```python
from build123d import *

# Parameters (mm, degrees)
ESQUISSE1_R        = 3.5
BOSS_EXTRU_1_DEPTH = 2
BOSS_EXTRU_2_START = 2
BOSS_EXTRU_2_DEPTH = 4
CONG_1_R           = 1


with BuildPart() as part:
    # Esquisse1 → Boss.-Extru.1 (new body)
    with BuildSketch(Plane.XY):
        with BuildLine():
            Line((8.486931566, 0), (59.535501901, 0))
            ThreePointArc((59.535501901, 0), (65.701431316, -2.44398639), (68.518594603, -8.448596789))
            Line((68.518594603, -8.448596789), (73.575299132, -90.829048435))
            ThreePointArc((73.575299132, -90.829048435), (76.596287018, -97.01955194), (83.109795045, -99.260737926))
            Line((83.109795045, -99.260737926), (85.106037868, -99.13820388))
            ThreePointArc((85.106037868, -99.13820388), (91.296541372, -96.117215994), (93.537727359, -89.603707966))
            Line((93.537727359, -89.603707966), (87.328590379, 11.551403211))
            ThreePointArc((87.328590379, 11.551403211), (84.511427092, 17.55601361), (78.345497677, 20))
            Line((78.345497677, 20), (-10.372916358, 20))
            ThreePointArc((-10.372916358, 20), (-16.547500996, 17.547862594), (-19.357434532, 11.527667678))
            Line((-19.357434532, 11.527667678), (-25.311005353, -89.842886985))
            ThreePointArc((-25.311005353, -89.842886985), (-23.052618299, -96.350450996), (-16.854154857, -99.355072837))
            Line((-16.854154857, -99.355072837), (-14.857595263, -99.472332322))
            ThreePointArc((-14.857595263, -99.472332322), (-8.350031252, -97.213945268), (-5.34540941, -91.015481826))
            Line((-5.34540941, -91.015481826), (-0.497586608, -8.472332322))
            ThreePointArc((-0.497586608, -8.472332322), (2.312346928, -2.452137406), (8.486931566, 0))
        make_face()
        with Locations((33.998753696, 10)):
            Circle(ESQUISSE1_R, mode=Mode.SUBTRACT)
    extrude(amount=BOSS_EXTRU_1_DEPTH)

    # Esquisse1<4> → Boss.-Extru.2 (add)
    with BuildSketch(Plane.XY.offset(BOSS_EXTRU_2_START)):
        with BuildLine():
            Line((8.486931566, 0), (59.535501901, 0))
            ThreePointArc((59.535501901, 0), (65.701431316, -2.44398639), (68.518594603, -8.448596789))
            Line((68.518594603, -8.448596789), (73.575299132, -90.829048435))
            ThreePointArc((73.575299132, -90.829048435), (76.596287018, -97.01955194), (83.109795045, -99.260737926))
            Line((83.109795045, -99.260737926), (85.106037868, -99.13820388))
            ThreePointArc((85.106037868, -99.13820388), (91.296541372, -96.117215994), (93.537727359, -89.603707966))
            Line((93.537727359, -89.603707966), (87.328590379, 11.551403211))
            ThreePointArc((87.328590379, 11.551403211), (84.511427092, 17.55601361), (78.345497677, 20))
            Line((78.345497677, 20), (-10.372916358, 20))
            ThreePointArc((-10.372916358, 20), (-16.547500996, 17.547862594), (-19.357434532, 11.527667678))
            Line((-19.357434532, 11.527667678), (-25.311005353, -89.842886985))
            ThreePointArc((-25.311005353, -89.842886985), (-23.052618299, -96.350450996), (-16.854154857, -99.355072837))
            Line((-16.854154857, -99.355072837), (-14.857595263, -99.472332322))
            ThreePointArc((-14.857595263, -99.472332322), (-8.350031252, -97.213945268), (-5.34540941, -91.015481826))
            Line((-5.34540941, -91.015481826), (-0.497586608, -8.472332322))
            ThreePointArc((-0.497586608, -8.472332322), (2.312346928, -2.452137406), (8.486931566, 0))
        make_face()
        with BuildLine():
            Line((-10.372916358, 18), (78.345497677, 18))
            ThreePointArc((78.345497677, 18), (83.141220555, 16.099121696), (85.332347556, 11.428869164))
            Line((85.332347556, 11.428869164), (91.541484536, -89.726242013))
            ThreePointArc((91.541484536, -89.726242013), (89.79833988, -94.792303812), (84.983503821, -97.141961057))
            Line((84.983503821, -97.141961057), (82.987260998, -97.264495104))
            ThreePointArc((82.987260998, -97.264495104), (77.921199199, -95.521350447), (75.571541954, -90.706514388))
            Line((75.571541954, -90.706514388), (70.514837426, -8.326062742))
            ThreePointArc((70.514837426, -8.326062742), (67.071637853, -0.987094477), (59.535501901, 2))
            Line((59.535501901, 2), (8.486931566, 2))
            ThreePointArc((8.486931566, 2), (0.940217009, -0.997056829), (-2.494146203, -8.355072837))
            Line((-2.494146203, -8.355072837), (-7.341969005, -90.898222342))
            ThreePointArc((-7.341969005, -90.898222342), (-9.678897103, -95.719249463), (-14.740335779, -97.475772727))
            Line((-14.740335779, -97.475772727), (-16.736895373, -97.358513243))
            ThreePointArc((-16.736895373, -97.358513243), (-21.557922495, -95.021585145), (-23.314445759, -89.960146469))
            Line((-23.314445759, -89.960146469), (-17.360874938, 11.410408194))
            ThreePointArc((-17.360874938, 11.410408194), (-15.175371076, 16.092782018), (-10.372916358, 18))
        make_face(mode=Mode.SUBTRACT)
    extrude(amount=BOSS_EXTRU_2_DEPTH)

    # Congé1
    cong_1_edges = [part.edges().sort_by_distance(p)[0] for p in [
        (-22.334219943, -39.157609653, 0),
        (-23.052618299, -96.350450996, 0),
        (-15.85587506, -99.41370258, 0),
        (-8.350031252, -97.213945268, 0),
        (-2.921498009, -49.743907074, 0),
        (2.312346928, -2.452137406, 0),
        (34.011216733, 0, 0),
        (65.701431316, -2.44398639, 0),
        (71.046946867, -49.638822612, 0),
        (76.596287018, -97.01955194, 0),
        (84.107916456, -99.199470903, 0),
        (91.296541372, -96.117215994, 0),
        (90.433158869, -39.026152378, 0),
        (84.511427092, 17.55601361, 0),
        (33.986290659, 20, 0),
        (-16.547500996, 17.547862594, 0),
    ]]
    fillet(cong_1_edges, radius=CONG_1_R)


solid = part.part
```
Input: part model. Units: mm. Frame: model coordinates. A direction names the side the tool comes from. Coordinates: 2 decimals unless noted, no trailing zeros. Loops run counter-clockwise (first coordinate to the right, second up) from the corner with the lowest first, then second, coordinate; pieces in that order, holes last.
Q1. Line query: line 1 along X through (y, z) = (-61, 4.5); line 2 along Y through (x, z) = (32, 5.5); line 3 along X through (y, z) = (-71, 4.5). Output: solid intervals per line, ascending.
Results are:
line 1: x = -23.62 to -21.61, -5.59 to -3.58, 71.74 to 73.75, 89.78 to 91.78
line 2: y = 0 to 2, 18 to 20
line 3: x = -24.2 to -22.2, -6.17 to -4.17, 72.36 to 74.36, 90.39 to 92.4
Q2. Mould query, pull axis Y, two halves, no side actions, for faces 4 (the flat face through (34, 0, 3)), 5 (the cylindrical face through (90.1, -38.3, 0.3)), 6 (the cylindrical face through (89.849, -94.734, 3.972)). Classes: +Y half, -Y half, draft (parallel to the pull), parting line (faces both ways), or undercut.
Results are:
face 4: -Y half
face 5: +Y half
face 6: undercut
Q3. Section A-A, the plane x = 34.5. Return the cut outline in (y, z).
Results are:
outline: (0, 1) arc R1 ccw to (1, 0) - (6.54, 0) - (6.54, 2) - (2, 2) - (2, 6) - (0, 6) - close; (13.46, 0) - (19, 0) arc R1 ccw to (20, 1) - (20, 6) - (18, 6) - (18, 2) - (13.46, 2) - close
Q4. Contact query for a flat-ended pin moving along its axis: pin 1 (1.2 mm diameter, centred on x = 27, z = 3.5, fed in from -Y). Output: stop coordinate, or through.
Results are:
pin 1: stops at y = 0
Q5. Set-up query: faces 1 (the flat face through (88.393, -38.441, 3.972)), 2 (the cylindrical face through (-3.188, -49.148, 0.285)), 3 (the cylindrical face through (76.52, -96.95, 3.46)). Return all of +Z, -Z, +X, -X, +Y, -Y with unobstructed straight access to the full face (end or side cutting, diameter ignored); none if empty.
Results are:
face 1: +Z
face 2: -Z, -Y
face 3: +Z, -Z, -Y
Q6. Section B-B, the plane x = 11.5. Return the cut outline in (y, z).
Results are:
outline: (0, 1) arc R1 ccw to (1, 0) - (19, 0) arc R1 ccw to (20, 1) - (20, 6) - (18, 6) - (18, 2) - (2, 2) - (2, 6) - (0, 6) - close
